Check sheet for the modelled part. Datum: model origin and axes. Units: mm. Face numbers are marked on the shaded views. Give positions to 0.01 mm unless a question says otherwise; leave off trailing zeros. Order: outer loops, then holes, each group sorted by start corner. A loop starts at its lowest first (then second) coordinate and runs counter-clockwise, first axis right, second up. Notation, with made-up numbers: (50, -15.75) - (69, -15.75) arc R8 cw to (69, -7.75) - close; hole circle Ø9 at (-16.5, -27). An arc over 180 degrees is marked (long way). Answer in a Markdown table with one row per item.
from build123d import *

# Parameters (mm, degrees)
F1_DEPTH = 9.525
F2_W     = 12.7
F2_H     = 241.3
F3_DEPTH = 25.4
F6_DEPTH = 25.4


with BuildPart() as f1:
    # F0 (on Right) → F1 (new body)
    with BuildSketch(Plane.YZ):
        with BuildLine():
            Line((29.845, -31.75), (0, -31.75))
            Line((0, -31.75), (0, -273.05))
            Line((0, -273.05), (29.845, -273.05))
            ThreePointArc((29.845, -273.05), (31.192038, -273.607962), (31.75, -274.955))
            Line((31.75, -274.955), (31.75, -304.8))
            Line((31.75, -304.8), (62.456746, -304.8))
            ThreePointArc((62.456746, -304.8), (112.216851, -175.710639), (222.25, -91.848627))
            Line((222.25, -91.848627), (222.25, -64.650771))
            ThreePointArc((222.25, -64.650771), (218.132973, -55.290078), (208.45117, -51.998397))
            Line((208.45117, -51.998397), (178.380117, -54.61))
            Line((178.380117, -54.61), (158.75, -63.5))
            Line((158.75, -63.5), (107.95, -63.5))
            Line((107.95, -63.5), (107.95, -38.1))
            ThreePointArc((107.95, -38.1), (111.669744, -29.119744), (120.65, -25.4))
            Line((120.65, -25.4), (209.55, -25.4))
            ThreePointArc((209.55, -25.4), (218.530256, -21.680256), (222.25, -12.7))
            ThreePointArc((222.25, -12.7), (218.530256, -3.719744), (209.55, 0))
            Line((209.55, 0), (31.75, 0))
            Line((31.75, 0), (31.75, -29.845))
            ThreePointArc((31.75, -29.845), (31.192038, -31.192038), (29.845, -31.75))
        make_face()
    extrude(amount=F1_DEPTH)

    # F2 (on face) → F3 (cut)
    with BuildSketch(Plane.YZ.offset(9.525)):
        with Locations((6.35, -152.4)):
            Rectangle(F2_W, F2_H)
    extrude(amount=-F3_DEPTH, mode=Mode.SUBTRACT)

    # F4: F1 across face


with BuildPart() as f1_1:
    add(f1.part)
    add(f1.part.mirror(Plane(origin=(4.7625, 12.7, -152.4), x_dir=(1, 0, 0), z_dir=(0, -1, 0))))

    # F5 (on face) → F6 (cut)
    with BuildSketch(Plane.YZ.offset(9.525)):
        with BuildLine():
            Line((32.146875, 0), (-6.746875, 0))
            Line((-6.746875, 0), (-6.746875, -29.845))
            ThreePointArc((-6.746875, -29.845), (-6.188913, -31.192038), (-4.841875, -31.75))
            Line((-4.841875, -31.75), (30.241875, -31.75))
            ThreePointArc((30.241875, -31.75), (31.588913, -31.192038), (32.146875, -29.845))
            Line((32.146875, -29.845), (32.146875, 0))
        make_face()
        with BuildLine():
            Line((-6.746875, -274.955), (-6.746875, -304.8))
            Line((-6.746875, -304.8), (32.146875, -304.8))
            Line((32.146875, -304.8), (32.146875, -274.955))
            ThreePointArc((32.146875, -274.955), (31.588913, -273.607962), (30.241875, -273.05))
            Line((30.241875, -273.05), (-4.841875, -273.05))
            ThreePointArc((-4.841875, -273.05), (-6.188913, -273.607962), (-6.746875, -274.955))
        make_face()
    extrude(amount=-F6_DEPTH, mode=Mode.SUBTRACT)


solid = f1_1.part
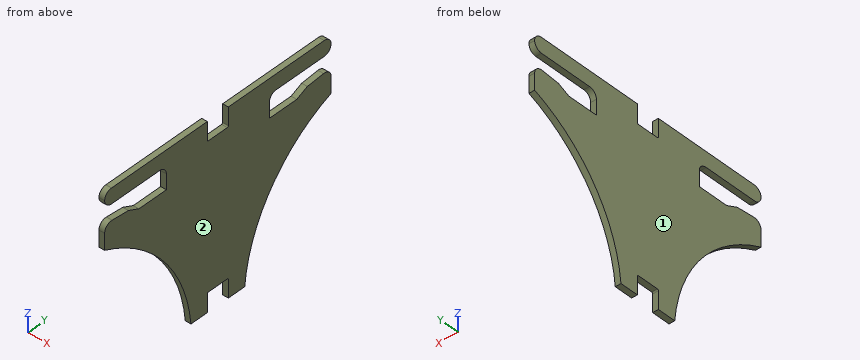
(1) Thickness scan on L1, parallel to Y at x = 2, z = -60; L2, parallel to Y at x = 6.75, z = -284; L3, parallel to Z at x = 9, y = 140.5. Record the ranges inside material, lowest first.
Geometry says:
| item | result |
|---|---|
| L1 | -195.97 to -141.08, -82.55 to 107.95, 166.48 to 221.37 |
| L2 | -39.85 to -6.75, 32.15 to 65.25 |
| L3 | -143.95 to -63.5, -25.4 to 0 |
(2) Cross-section at B-B, the plane y = 114.5. Record the cut outline in (x, z) (1 decimal).
Geometry says:
| item | result |
|---|---|
| outline | (0, -172.7) - (9.5, -172.7) - (9.5, -63.5) - (0, -63.5) - close; (0, -27) - (9.5, -27) - (9.5, 0) - (0, 0) - close |
(3) Mould release check, pull along X, two halves, no side actions. Record for the marked faces 1 and 2: pulls with the +X half, pulls with the -X half, needs draft (parallel to the pull), parting line crosses it, or undercut.
Geometry says:
| item | result |
|---|---|
| face 1 | pulls with the -X half |
| face 2 | pulls with the +X half |
(4) Cross-section at A-A, the plane z = -282. Record the cut outline in (x, y) (3 decimals).
Geometry says:
| item | result |
|---|---|
| outline | (0, -40.21) - (9.525, -40.21) - (9.525, -6.747) - (0, -6.747) - close; (0, 32.147) - (9.525, 32.147) - (9.525, 65.61) - (0, 65.61) - close |
(5) Gauge pin test, flat ends, axial feed: P1, Ø3, axis at x = 3, z = -287, coming from the -Y side; P2, Ø3, axis at x = 2.5, z = -57, coming from the +Y side; P3, Ø3, axis at x = 4.5, z = -285.5, coming from the +Y side. Record the tip position at first contact, or that the pin passes through.
Geometry says:
| item | result |
|---|---|
| P1 | y = -39.59 |
| P2 | y = 220.66 |
| P3 | y = 65.25 |
(6) Cross-section at D-D, the plane z = -200. Record the cut outline in (x, y) (3 decimals), then the cut area to 3 significant figures.
Geometry says:
| item | result |
|---|---|
| outline | (0, -70.683) - (9.525, -70.683) - (9.525, 96.083) - (0, 96.083) - close |
| area | 1,590 mm² |
(7) Cross-section at C-C, the plane y = 14. Record the cut outline in (x, z) (3 decimals).
Geometry says:
| item | result |
|---|---|
| outline | (0, -273.05) - (9.525, -273.05) - (9.525, -31.75) - (0, -31.75) - close |
